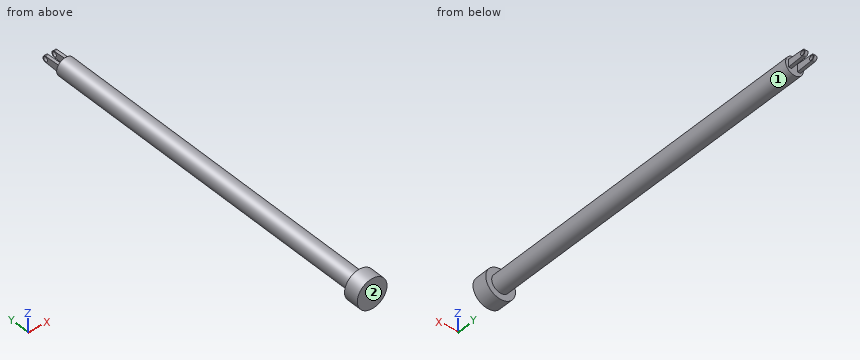
```python
from build123d import *

# Parameters (mm, degrees)
SKETCH1_W           = 3
SKETCH1_H           = 10
SKETCH2_W           = 1
SKETCH2_H           = 2.5
BOSS_EXTRUDE2_DEPTH = 7
SKETCH3_R           = 0.75
CUT_EXTRUDE1_DEPTH  = 7


with BuildPart() as part:
    # Sketch1 → Revolve1 (revolve)
    with BuildSketch(Plane.XY, mode=Mode.PRIVATE) as revolve1_sk:
        Polygon((3, 110), (0, 110), (0, 0), (5, 0), (5, 5), (3, 5), align=None)
        with Locations((1.5, 115)):
            Rectangle(SKETCH1_W, SKETCH1_H)
    revolve(revolve1_sk.sketch.rotate(Axis((0, 0, 0), (0, 1, 0)), 90), axis=Axis((0, 0, 0), (0, 1, 0)))

    # Sketch2 → Boss-Extrude2 (add)
    with BuildSketch(Plane(origin=(0, 120, 0), x_dir=(1, 0, 0), z_dir=(0, 1, 0))):
        with Locations((-1.5, 0)):
            Rectangle(SKETCH2_W, SKETCH2_H)
        with Locations((1.5, 0)):
            Rectangle(SKETCH2_W, SKETCH2_H)
    extrude(amount=BOSS_EXTRUDE2_DEPTH)

    # Sketch3 → Cut-Extrude1 (cut)
    with BuildSketch(Plane.ZY.offset(2)):
        with Locations(Location((0, 125.5, 0), (0, 0, 180))):
            Circle(SKETCH3_R)
        with BuildLine():
            Line((1.25, 120), (0.99897696, 125.545222036))
            ThreePointArc((0.99897696, 125.545222036), (0, 126.5), (-0.99897696, 125.545222036))
            Line((-0.99897696, 125.545222036), (-1.25, 120))
            Line((-1.25, 120), (-1.25, 127))
            Line((-1.25, 127), (1.25, 127))
            Line((1.25, 127), (1.25, 120))
        make_face()
    extrude(amount=-CUT_EXTRUDE1_DEPTH, mode=Mode.SUBTRACT)


solid = part.part
```
Geometry check sheet. Reference: the model listing, model coordinates, mm. Face numbers are marked on the shaded views. A direction names the side the tool comes from. Coordinates: 2 decimals unless noted, no trailing zeros. Order: outer loops, then holes, each group sorted by start corner. A loop starts at its lowest first (then second) coordinate and runs counter-clockwise, first axis right, second up. Notation, with made-up numbers: (-19.75, 0) - (13.25, 0) arc R26 ccw to (13.25, 39) - close; hole circle Ø6 at (68, 2.5). An arc over 180 degrees is marked (long way). Use one line per item in the form item = value.
1. Access from +Z, -Z, +X, -X, +Y, -Y to the whole of each face (thin tool, end or side, straight path). Record for the marked faces 1 and 2.
Here are the results:
face_1 = +Y
face_2 = +Z, -Z, +X, -X, -Y
2. Section check A-A (y = 99.5). Record the boundary of the cut face in (x, z), then the cut area to 3 significant figures.
Here are the results:
outline = circle Ø6 at (0, 0)
area = 28.3 mm²
3. Gauge pin test, flat ends, axial feed: pin 1 (1.5 mm diameter, centred on x = -1, y = 111.5, fed in from +Z); pin 2 (5 mm diameter, centred on y = 105.5, z = 1.5, fed in from +X); pin 3 (0.8 mm diameter, centred on y = 124, z = -0.5, fed in from +X); pin 4 (3 mm diameter, centred on x = 1, z = -1, fed in from +Y). Record the tip position at first contact, or that the pin passes through.
Here are the results:
pin_1 = 2.99
pin_2 = 3
pin_3 = 2
pin_4 = 126.5
4. Scan lines: line 1 (Z direction, x = 1.5, y = 125.5); line 2 (Y direction, x = 0.75, z = -3); line 3 (Y direction, x = 0, z = 1). Record each from-to range of solid material in increasing order.
Here are the results:
line_1 = -1 to -0.75, 0.75 to 1
line_2 = 0 to 5
line_3 = 0 to 120
